The figure shows three views and two pictorial views of one solid part (mm, origin at its lowest corner). Answer the questions. Round coordinates to 2 decimals unless told otherwise and drop trailing zeros. Order: outer loops, then holes, each group sorted by start corner. A loop starts at its lowest first (then second) coordinate and runs counter-clockwise, first axis right, second up. Notation, with made-up numbers: M 66,28.25 L 107,28.25 A28 ccw 107,48.25 Z; hole C 82.5,57 d4. An arc over 180 degrees is marked long. Answer as CSV lines item,"result".
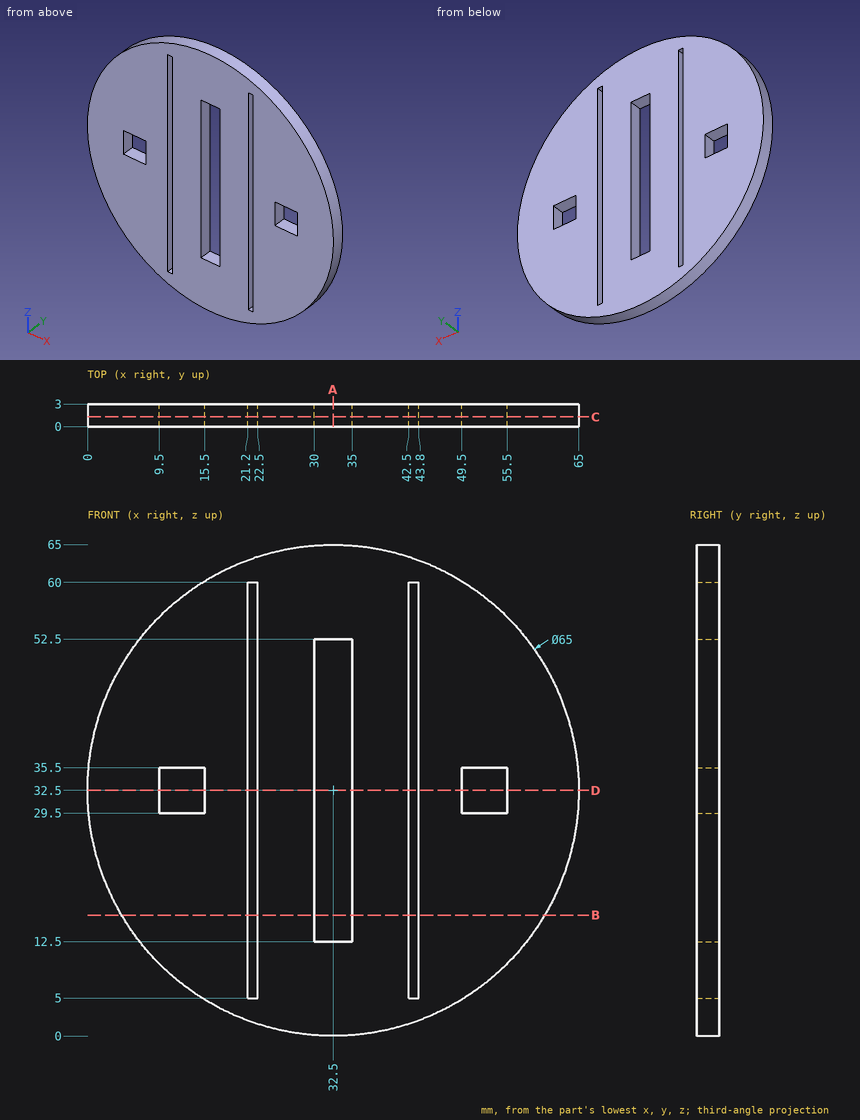
Item 1: Find the intervals of material crossed by probe 1 along X at (y, z) = (2.3, 32); probe 2 along X at (y, z) = (0.95, 24.5); probe 3 along X at (y, z) = (0.25, 30.5), in increasing order. Write a range as [from, to].
Ans:
probe 1,"[0, 9.5], [15.5, 21.2], [22.5, 30], [35, 42.5], [43.8, 49.5], [55.5, 65]"
probe 2,"[1, 21.2], [22.5, 30], [35, 42.5], [43.8, 64]"
probe 3,"[0.06, 9.5], [15.5, 21.2], [22.5, 30], [35, 42.5], [43.8, 49.5], [55.5, 64.94]"
Item 2: Flat-ended cylindrical pins translate along their axes: pin 1 (1.5 mm diameter, centred on x = 56.5, y = 2, fed in from +Z); pin 2 (1.4 mm diameter, centred on x = 21.5, y = 1, fed in from -Z); pin 3 (0.9 mm diameter, centred on y = 1.5, z = 28.5, fed in from -X). Find the tip coordinate at first contact, or state that the pin passes through.
Ans:
pin 1,"z = 55.21"
pin 2,"z = 1.68"
pin 3,"x = 0.19"
Item 3: A cutting plane is placed at A-A, the plane x = 32.5. Determine the outline of the cut face in (y, z).
Ans:
outline,"M 0,0 L 3,0 L 3,12.5 L 0,12.5 Z; M 0,52.5 L 3,52.5 L 3,65 L 0,65 Z"
Item 4: A cutting plane is placed at D-D, the plane z = 32.5. Determine the outline of the cut face in (x, y).
Ans:
outline,"M 0,0 L 9.5,0 L 9.5,3 L 0,3 Z; M 15.5,0 L 21.2,0 L 21.2,3 L 15.5,3 Z; M 22.5,0 L 30,0 L 30,3 L 22.5,3 Z; M 35,0 L 42.5,0 L 42.5,3 L 35,3 Z; M 43.8,0 L 49.5,0 L 49.5,3 L 43.8,3 Z; M 55.5,0 L 65,0 L 65,3 L 55.5,3 Z"
Item 5: A cutting plane is placed at C-C, the plane y = 1.3. Determine the outline of the cut face in (x, z), and give its area (3 significant figures).
Ans:
outline,"C 32.5,32.5 d65; hole M 9.5,29.5 L 15.5,29.5 L 15.5,35.5 L 9.5,35.5 Z; hole M 21.2,5 L 22.5,5 L 22.5,60 L 21.2,60 Z; hole M 30,12.5 L 35,12.5 L 35,52.5 L 30,52.5 Z; hole M 42.5,5 L 43.8,5 L 43.8,60 L 42.5,60 Z; hole M 49.5,29.5 L 55.5,29.5 L 55.5,35.5 L 49.5,35.5 Z"
area,"2,900 mm2"
Item 6: A cutting plane is placed at B-B, the plane z = 16. Determine the outline of the cut face in (x, y).
Ans:
outline,"M 4.5,0 L 21.2,0 L 21.2,3 L 4.5,3 Z; M 22.5,0 L 30,0 L 30,3 L 22.5,3 Z; M 35,0 L 42.5,0 L 42.5,3 L 35,3 Z; M 43.8,0 L 60.5,0 L 60.5,3 L 43.8,3 Z"
